from build123d import *

# Parameters (mm, degrees)
F0_W     = 12.7
F0_H     = 4.7752
F2_R     = 2.3622
F3_R     = 4.7625
F4_DEPTH = 3.175
F5_R     = 2.3876
F6_DEPTH = 9.525


with BuildPart() as f1:
    # F0 (on Front) → F1 (revolve)
    with BuildSketch(Plane.XZ):
        with Locations((15.7442009076, 3.3685917145)):
            Rectangle(F0_W, F0_H)
    revolve(axis=Axis((9.3942009076, 0, 3.3685917145), (0, 0, -1)))

    # F2
    f2_edges = [f1.edges().sort_by_distance(p)[0] for p in [
        (-3.305799, 0, 5.756192),
        (-3.305799, 0, 0.980992),
    ]]
    fillet(f2_edges, radius=F2_R)

    # F3 (on face) → F4 (join)
    with BuildSketch(Plane.XY.offset(5.7561917145)):
        with Locations((9.3942009076, 0)):
            Circle(F3_R)
    extrude(amount=F4_DEPTH)

    # F5 (on face) → F6 (join)
    with BuildSketch(Plane.XY.offset(5.7561917145)):
        with Locations((9.3942009076, 0)):
            Circle(F5_R)
    extrude(amount=F6_DEPTH)


solid = f1.part
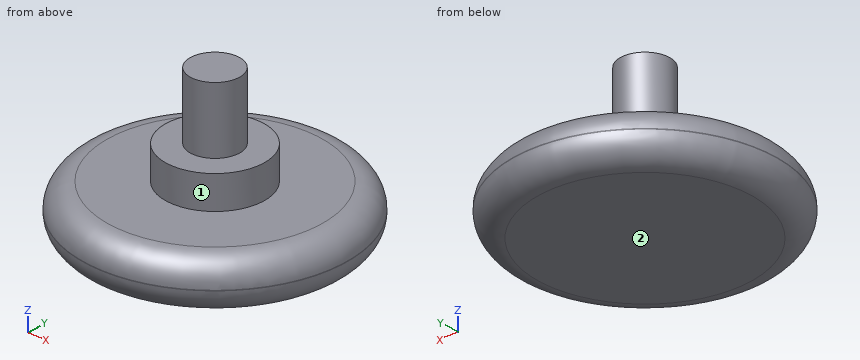
Source: CAD feature listing. Evaluate the final solid. Frame: model axes, mm. Face numbers are marked on the shaded views. A direction names the side the tool comes from. Give positions to 0.01 mm unless a question says otherwise; leave off trailing zeros. Write each loop counter-clockwise with the first axis right and the second up, starting at its lowest first coordinate (ties: lowest second). Pieces come first, ordered by that corner, then holes. Notation, with made-up numbers: (13, 87.25) -> (45, 87.25) arc R11 cw to (45, 97.25) -> close; hole circle Ø1 at (51.5, -25). An arc over 180 degrees is marked (long way). Write item = value, one per line.
Q1. Cut plane A-A on y = 0. Return loops of the section in (x, z), then the cut area to 3 significant figures.
Here are the results:
outline = (-3.31, 3.34) arc R2.36 ccw to (-0.94, 0.98) -> (19.73, 0.98) arc R2.36 ccw to (22.09, 3.34) -> (22.09, 3.39) arc R2.36 ccw to (19.73, 5.76) -> (14.16, 5.76) -> (14.16, 8.93) -> (11.78, 8.93) -> (11.78, 15.28) -> (7.01, 15.28) -> (7.01, 8.93) -> (4.63, 8.93) -> (4.63, 5.76) -> (-0.94, 5.76) arc R2.36 ccw to (-3.31, 3.39) -> close
area = 177 mm²
Q2. Cut plane C-C on z = 7.75. Return loops of the section in (x, y) (1 decimal), then the cut area to 3 significant figures.
Here are the results:
outline = circle Ø9.5 at (9.4, 0)
area = 71.3 mm²
Q3. Reachability of the marked faces 1 and 2 from +Z, -Z, +X, -X, +Y, -Y: full face, straight path, thin tool, end or side. Return the list, or none.
Here are the results:
face_1 = +Z
face_2 = -Z, +X, -X, +Y, -Y
Q4. Line query: line 1 (Y direction, x = 9.5, z = 6.5); line 2 (Y direction, x = 9.5, z = 13.25); line 3 (Z direction, x = 5.5, y = -8.75). Output: solid intervals per line, ascending. Write a range as from..to.
Here are the results:
line_1 = -4.76..4.76
line_2 = -2.39..2.39
line_3 = 0.98..5.76
Q5. First-contact query: pin 1 (3 mm diameter, centred on x = 19, y = -8.5, fed in from -Z); pin 2 (6 mm diameter, centred on y = -10, z = 3, fed in from +X); pin 3 (5 mm diameter, centred on x = 11, y = 2, fed in from +Z); pin 4 (4 mm diameter, centred on x = 2, z = 8, fed in from -Y). Flat tips, straight axial feed; report the tip coordinate or a pass-through.
Here are the results:
pin_1 = 1.2
pin_2 = 19.98
pin_3 = 15.28
pin_4 = through
Q6. Cut plane B-B on z = 9.75. Return loops of the section in (x, y).
Here are the results:
outline = circle Ø4.78 at (9.39, 0)
